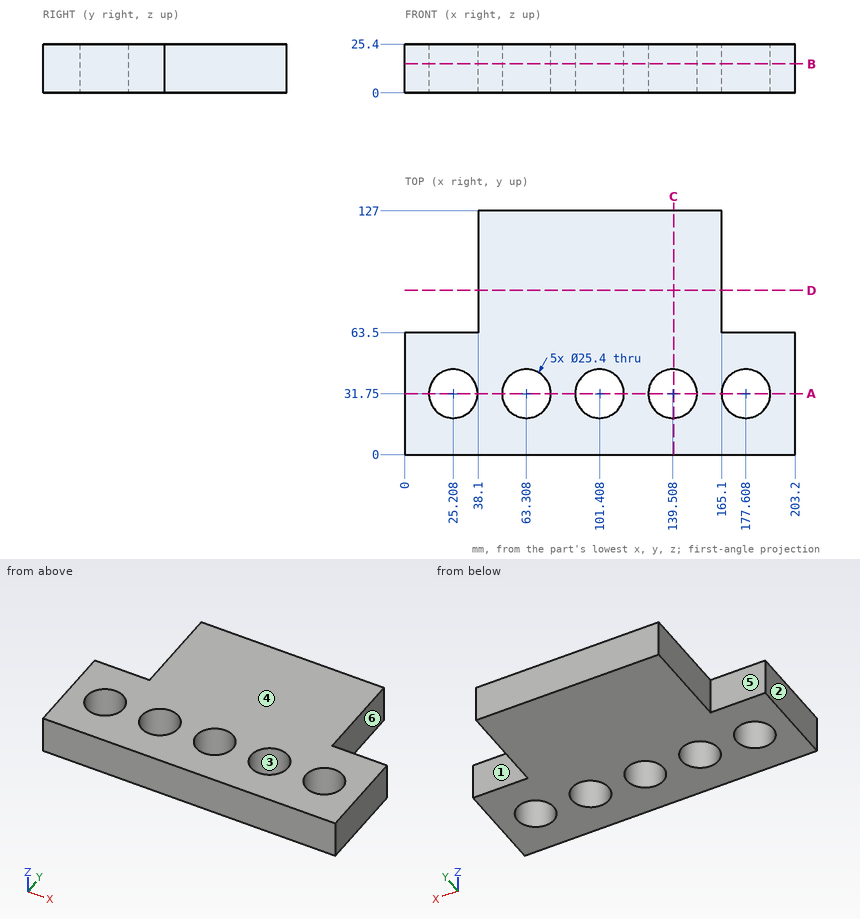
Geometry: see drawing. Coordinates: mm, zero at the bounding-box minimum. A direction names the side the tool comes from. Give positions to 0.01 mm unless a question says otherwise; leave off trailing zeros. Write each loop counter-clockwise with the first axis right and the second up, starting at its lowest first coordinate (ties: lowest second). Pieces come first, ordered by that corner, then holes. Notation, with made-up numbers: M 16.25,-3.5 L 59.25,-3.5 A16 ccw 59.25,17.5 Z; hole C 53,76 d7. An arc over 180 degrees is marked long. Answer in a Markdown table with one row per item. Add a question column.
(1) Section C-C on x = 140. Return loops of the section in (y, z), and give its area (3 significant figures).
(2) Section A-A on y = 31.75. Return loops of the section in (x, z).
(3) Reachability of the marked faces 4, 5 and 6 from +Z, -Z, +X, -X, +Y, -Y: full face, straight path, thin tool, end or side. Return the list, or none.
(4) Mould query, pull axis X, two halves, no side actions, for the marked faces 1, 2 and 3. Classes: +X half, -X half, draft (parallel to the pull), parting line (faces both ways), or undercut.
(5) Section B-B on z = 15. Return loops of the section in (x, y).
(6) First-contact query: pin 1 (7.5 mm diameter, centred on x = 13.5, z = 16, fed in from +Y); pin 2 (10 mm diameter, centred on y = 82.5, z = 19, fed in from -X). Flat tips, straight axial feed; report the tip coordinate or a pass-through.
(7) Section D-D on y = 85.5. Return loops of the section in (x, z).
(8) Ray query, line 1 (Y direction, x = 38, z = 14.25); line 2 (Y direction, x = 171.5, z = 18.5) (1 decimal); line 3 (X direction, y = 75.5, z = 22). Return the intervals inside material, ascending.
Result set:
| question | item | result |
|---|---|---|
| 1 | outline | M 0,0 L 19.06,0 L 19.06,25.4 L 0,25.4 Z; M 44.44,0 L 127,0 L 127,25.4 L 44.44,25.4 Z |
| 1 | area | 2,580 mm^2 |
| 2 | outline | M 0,0 L 12.51,0 L 12.51,25.4 L 0,25.4 Z; M 37.91,0 L 50.61,0 L 50.61,25.4 L 37.91,25.4 Z; M 76.01,0 L 88.71,0 L 88.71,25.4 L 76.01,25.4 Z; M 114.11,0 L 126.81,0 L 126.81,25.4 L 114.11,25.4 Z; M 152.21,0 L 164.91,0 L 164.91,25.4 L 152.21,25.4 Z; M 190.31,0 L 203.2,0 L 203.2,25.4 L 190.31,25.4 Z |
| 3 | face 4 | +Z, +X, -X, +Y, -Y |
| 3 | face 5 | +Z, -Z, -X, +Y |
| 3 | face 6 | +Z, -Z, +X, +Y |
| 4 | face 1 | draft |
| 4 | face 2 | -X half |
| 4 | face 3 | undercut |
| 5 | outline | M 0,0 L 203.2,0 L 203.2,63.5 L 165.1,63.5 L 165.1,127 L 38.1,127 L 38.1,63.5 L 0,63.5 Z; hole C 25.21,31.75 d25.4; hole C 63.31,31.75 d25.4; hole C 101.41,31.75 d25.4; hole C 139.51,31.75 d25.4; hole C 177.61,31.75 d25.4 |
| 6 | pin 1 | stops at y = 63.5 |
| 6 | pin 2 | stops at x = 38.1 |
| 7 | outline | M 38.1,0 L 165.1,0 L 165.1,25.4 L 38.1,25.4 Z |
| 8 | line 1 | y = 0 to 63.5 |
| 8 | line 2 | y = 0 to 20.6, 42.9 to 63.5 |
| 8 | line 3 | x = 38.1 to 165.1 |
